from build123d import *

# Parameters (mm, degrees)
BOSS_EXTRUDE1_DEPTH   = 30
CUT_EXTRUDE1_START    = -7.5
SKETCH3_W             = 34
SKETCH3_H             = 26
CUT_EXTRUDE1_DEPTH    = 35
F_4_0MM_DOWEL_HOLE2_D = 4.1
F_4_0MM_DOWEL_HOLE1_D = 4.1
BOSS_EXTRUDE2_DEPTH   = 4
BOSS_EXTRUDE3_DEPTH   = 10
F_4_0MM_DOWEL_HOLE3_D = 4.1


with BuildPart() as part:
    # Sketch1 → Boss-Extrude1 (new body)
    with BuildSketch(Plane(origin=(0, 0, 0), x_dir=(1, 0, 0), z_dir=(0, 1, 0))):
        with BuildLine():
            Line((42, 0), (42, 50))
            Line((42, 50), (4, 50))
            ThreePointArc((4, 50), (1.171572875, 48.828427125), (0, 46))
            Line((0, 46), (0, 4))
            ThreePointArc((0, 4), (1.171572875, 1.171572875), (4, 0))
            Line((4, 0), (42, 0))
        make_face()
    extrude(amount=BOSS_EXTRUDE1_DEPTH)

    # Sketch3 → Cut-Extrude1 (cut)
    with BuildSketch(Plane.XY.offset(CUT_EXTRUDE1_START)):
        with Locations((17, 17)):
            Rectangle(SKETCH3_W, SKETCH3_H)
    extrude(amount=-CUT_EXTRUDE1_DEPTH, mode=Mode.SUBTRACT)

    # Ø4.0mm Dowel Hole2 (through all)
    with Locations(Plane(origin=(25, 4, -35), x_dir=(1, 0, 0), z_dir=(0, 1, 0))):
        with Locations((0, 0), (0, -10), (0, -20), (-10, -10)):
            Hole(F_4_0MM_DOWEL_HOLE2_D / 2)

    # Ø4.0mm Dowel Hole1 (through all)
    with Locations(Plane(origin=(42, 23.5, -16.25), x_dir=(0, 0, 1), z_dir=(1, 0, 0))):
        with Locations((0, 0), (-17.5, 0), (-17.5, 13), (0, 13)):
            Hole(F_4_0MM_DOWEL_HOLE1_D / 2)

    # Sketch5 → Boss-Extrude2 (add)
    with BuildSketch(Plane(origin=(0, 30, 0), x_dir=(1, 0, 0), z_dir=(0, 1, 0))):
        with BuildLine():
            Line((4, 0), (46, 0))
            ThreePointArc((46, 0), (48.828427125, 1.171572875), (50, 4))
            Line((50, 4), (50, 46))
            ThreePointArc((50, 46), (48.828427125, 48.828427125), (46, 50))
            Line((46, 50), (4, 50))
            ThreePointArc((4, 50), (1.171572875, 48.828427125), (0, 46))
            Line((0, 46), (0, 4))
            ThreePointArc((0, 4), (1.171572875, 1.171572875), (4, 0))
        make_face()
    extrude(amount=BOSS_EXTRUDE2_DEPTH)

    # Sketch8 → Boss-Extrude3 (add)
    with BuildSketch(Plane(origin=(0, 34, 0), x_dir=(1, 0, 0), z_dir=(0, 1, 0))):
        with BuildLine():
            ThreePointArc((48, 25), (27.515082566, 47.862072515), (2.550055679, 30))
            Line((2.550055679, 30), (4.603921946, 30))
            ThreePointArc((4.603921946, 30), (27.518170056, 45.848472835), (46, 25))
            ThreePointArc((46, 25), (27.518170056, 4.151527165), (4.603921946, 20))
            Line((4.603921946, 20), (2.550055679, 20))
            ThreePointArc((2.550055679, 20), (27.515082566, 2.137927485), (48, 25))
        make_face()
    extrude(amount=BOSS_EXTRUDE3_DEPTH)

    # Ø4.0mm Dowel Hole3 (through all)
    with Locations(Plane(origin=(25, 44, -25), x_dir=(0, 0, 1), z_dir=(0, 1, 0))):
        with Locations((0, 0)):
            Hole(F_4_0MM_DOWEL_HOLE3_D / 2)


solid = part.part
Geometry: final body of the model. Coordinates: model frame, mm. A direction names the side the tool comes from. Give positions to 0.01 mm unless a question says otherwise; leave off trailing zeros. Write each loop counter-clockwise with the first axis right and the second up, starting at its lowest first coordinate (ties: lowest second). Pieces come first, ordered by that corner, then holes. Notation, with made-up numbers: (66.5, -10) -> (82.5, -10) arc R33 ccw to (82.5, 26) -> close; hole circle Ø8 at (-18.75, -3). An arc over 180 degrees is marked (long way). Answer in a Markdown table with one row per item.
(1) Section query D-D on z = -5.5. Return loops of the section in (x, y), then the cut area to 3 significant figures.
Answers below:
| item | result |
|---|---|
| outline | (0, 0) -> (42, 0) -> (42, 30) -> (50, 30) -> (50, 34) -> (37.2, 34) -> (37.2, 44) -> (32.79, 44) -> (32.79, 34) -> (17.21, 34) -> (17.21, 44) -> (12.8, 44) -> (12.8, 34) -> (0, 34) -> close |
| area | 1,550 mm^2 |
(2) Section query A-A on y = 23.5. Return loops of the section in (x, z).
Answers below:
| item | result |
|---|---|
| outline | (0, -46) arc R4 ccw to (4, -50) -> (42, -50) -> (42, -35.8) -> (34, -35.8) -> (34, -42.5) -> (0, -42.5) -> close; (0, -7.5) -> (34, -7.5) -> (34, -14.2) -> (42, -14.2) -> (42, 0) -> (4, 0) arc R4 ccw to (0, -4) -> close; (34, -31.7) -> (42, -31.7) -> (42, -18.3) -> (34, -18.3) -> close |
(3) Ray query, line 1 along Z through (x, y) = (38, 10.5); line 2 along Y through (x, z) = (38.75, -16.25); line 3 along Y through (x, z) = (17.5, -18). Return the intervals inside material, ascending. Write a range as [from, to].
Answers below:
| item | result |
|---|---|
| line 1 | [-50, -35.8], [-31.7, -18.3], [-14.2, 0] |
| line 2 | [0, 8.45], [12.55, 21.45], [25.55, 34] |
| line 3 | [0, 4], [30, 34] |
(4) Section query B-B on x = 25. State how many separate pieces and enclosed holes the cut face has, then the cut area to 3 significant figures.
Answers below:
| item | result |
|---|---|
| separate pieces | 4 |
| enclosed holes | 0 |
| area | 764 mm^2 |
(5) Pin query (flat end, axial travel): pin 1 (4 mm diameter, centred on y = 26.5, z = -21.5, fed in from +X); pin 2 (4 mm diameter, centred on y = 23, z = -25.5, fed in from -X); pin 3 (4.5 mm diameter, centred on x = 15, z = -25, fed in from +Y). Return the tip coordinate at first contact, or that it passes through.
Answers below:
| item | result |
|---|---|
| pin 1 | x = 42 |
| pin 2 | x = 34 |
| pin 3 | y = 34 |
(6) Draft query along X for faces 1 (the flat face through (17, 17, -42.5)), 2 (the cylindrical face through (25.267, 1.972, -37.033)), 3 (the flat face through (34, 17, -25)). Return one class per face: +X half, -X half, draft (parallel to the pull), parting line (faces both ways), or undercut.
Answers below:
| item | result |
|---|---|
| face 1 | draft |
| face 2 | undercut |
| face 3 | -X half |
(7) Set-up query: faces 4 (the flat face through (4, 39, -30)), 5 (the flat face through (46, 30, -25)), 6 (the flat face through (17, 30, -25)), 7 (the cylindrical face through (25.444, 1.972, -12.999)), 8 (the cylindrical face through (37.944, 11.747, -14.623)). Return all of +Z, -Z, +X, -X, +Y, -Y with unobstructed straight access to the full face (end or side cutting, diameter ignored); none if empty.
Answers below:
| item | result |
|---|---|
| face 4 | -X, +Y |
| face 5 | +Z, -Z, +X, -Y |
| face 6 | -X |
| face 7 | -Y |
| face 8 | +X, -X |
